Input: part model. Units: mm. Frame: model coordinates. Face numbers are marked on the shaded views. A direction names the side the tool comes from. Give positions to 0.01 mm unless a question says otherwise; leave off trailing zeros. Write each loop counter-clockwise with the first axis right and the second up, starting at its lowest first coordinate (ties: lowest second). Pieces come first, ordered by that corner, then holes. Notation, with made-up numbers: (79, 59) - (107, 59) arc R10 ccw to (107, 72) - close; hole circle Ø4 at (24.25, 48.5). An arc over 180 degrees is marked (long way). Answer as CSV lines item,"result".
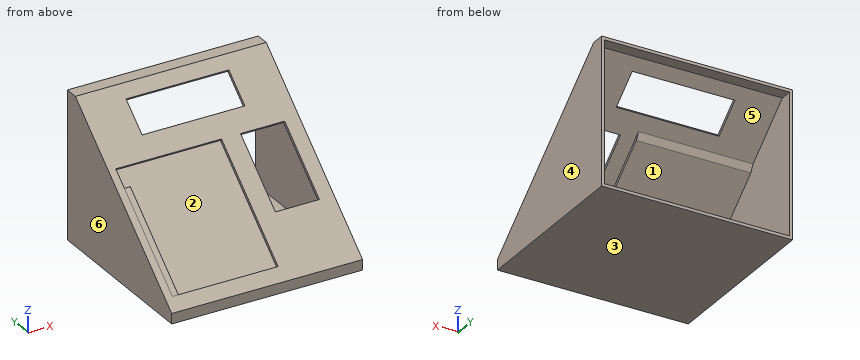
Solid Edge part; units mm, degrees
sketch "Sketch1" plane through (0, 0, 0) normal (0, 0, 1) x (1, 0, 0)
  line L0 (-65, -60) -> (65, -60)
  line L1 (65, -60) -> (65, 60)
  line L2 (65, 60) -> (-65, 60)
  line L3 (-65, 60) -> (-65, -60)
extrude "Protrusion1" add sketch "Sketch1" along normal blind 2
sketch "Sketch2" plane through (0, 0, 2) normal (0, 0, 1) x (1, 0, 0)
  line L0 (-65, -60) -> (-63, -60)
  line L1 (-63, -60) -> (-63, 60)
  line L2 (-63, 60) -> (-65, 60)
  line L3 (-65, 60) -> (-65, -60)
  line L4 (65, 60) -> (63, 60)
  line L5 (63, 60) -> (63, -60)
  line L6 (63, -60) -> (65, -60)
  line L7 (65, -60) -> (65, 60)
extrude "Protrusion2" add sketch "Sketch2" along normal blind 98
sketch "Sketch3" plane through (65, 0, 51) normal (1, 0, 0) x (0, 1, 0)
  line L0 (-60, 49) -> (-60, -44)
  line L1 (50.8331, 49) -> (-60, -44)
  line L2 (50.8331, 49) -> (-60, 49)
  dimension "D1" = 60
extrude "ExtrudedCutout_1" cut sketch "Sketch3" against normal blind 130
sketch "Sketch4" plane through (-63, 0, 52) normal (1, 0, 0) x (0, 1, 0)
  line L0 (-60, -45) -> (-60, -50)
  line L1 (-60, -50) -> (-58, -50)
  line L2 (-58, -50) -> (-58, -45.9326)
  line L3 (51.561, 46) -> (-58, -45.9326)
  line L4 (60, 46) -> (51.561, 46)
  line L5 (60, 48) -> (60, 46)
  line L6 (60, 48) -> (50.8331, 48)
  line L7 (50.8331, 48) -> (-60, -45)
extrude "Protrusion3" add sketch "Sketch4" along normal up to vertex (128 mm away)
sketch "Sketch5" plane through (0, -4.5835, 53.5) normal (0, -0.6427876, 0.7660444) x (1, 0, 0)
  line L0 (35, 62.3412) -> (-35, 62.3412)
  line L1 (-35, 62.3412) -> (-35, 38.3412)
  line L2 (-35, 38.3412) -> (35, 38.3412)
  line L3 (35, 38.3412) -> (35, 62.3412)
extrude "Cutout1" cut sketch "Sketch5" against normal blind 2
sketch "Sketch6" plane through (0, -4.5835, 53.5) normal (0, -0.6427876, 0.7660444) x (1, 0, 0)
  line L0 (-60, -62.3412) -> (12, -62.3412)
  line L1 (12, -62.3412) -> (12, 22.6588)
  line L2 (12, 22.6588) -> (-60, 22.6588)
  line L3 (-60, 22.6588) -> (-60, -62.3412)
  dimension "D1" = 12
  dimension "D2" = 12
extrude "ExtrudedCutout_3" cut sketch "Sketch6" against normal blind 2
sketch "Sketch7" plane through (0, -4.5835, 53.5) normal (0, -0.6427876, 0.7660444) x (1, 0, 0)
  line L0 (25, -29.5572) -> (55, -29.5572)
  line L1 (55, -29.5572) -> (55, 22.6588)
  line L2 (55, 22.6588) -> (25, 22.6588)
  line L3 (25, 22.6588) -> (25, -29.5572)
  dimension "D1" = 55
  dimension "D2" = 55
extrude "Cutout2" cut sketch "Sketch7" against normal blind 2
sketch "Sketch8" plane through (-63, 1, 50) normal (1, 0, 0) x (0, 1, 0)
  line L0 (14.3454, 15.0006) -> (-50.7684, -39.6363)
  line L1 (-55.8842, -41.3182) -> (-50.7684, -39.6363)
  line L2 (-52.054, -38.1042) -> (-55.8842, -41.3182)
  line L3 (-52.054, -38.1042) -> (13.0598, 16.5327)
  line L4 (13.0598, 16.5327) -> (16.89, 19.7467)
  line L5 (16.89, 19.7467) -> (14.3454, 15.0006)
extrude "ExtrudedProtrusion_6" add sketch "Sketch8" along normal blind 78
sketch "Sketch9" plane through (-60, -19.1399, 39.9803) normal (1, 0, 0) x (0, 0.7660444, 0.6427876)
  line L0 (-42.5, 1) -> (29.5, 1)
  line L1 (29.5, 1) -> (29.5, 0)
  line L2 (29.5, 0) -> (-42.5, 0)
  line L3 (-42.5, 0) -> (-42.5, 1)
extrude "ExtrudedProtrusion_7" add sketch "Sketch9" along normal blind 4
Item 1: Ray query, line 1 (X direction, y = 19.5, z = 47); line 2 (Z direction, x = -4, y = 54.5); line 3 (Z direction, x = -56, y = 20). Return the intervals inside material, ascending. Write a range as from..to.
The answers:
line 1,"-65..-63, 63..65"
line 2,"0..2, 98..100"
line 3,"0..2, 71.52..74.13"
Item 2: Mould query, pull axis X, two halves, no side actions, for the marked faces 1, 2, 3 and 4. Classes: +X half, -X half, draft (parallel to the pull), parting line (faces both ways), or undercut.
The answers:
face 1,"undercut"
face 2,"undercut"
face 3,"draft"
face 4,"+X half"
Item 3: Reachability of the marked faces 5 and 6 from +Z, -Z, +X, -X, +Y, -Y: full face, straight path, thin tool, end or side. Return the list, or none.
The answers:
face 5,"+Y"
face 6,"+Z, -Z, -X, +Y, -Y"
Item 4: Cut plane A-A on z = 90. Return the cut outline in (x, y).
The answers:
outline,"(-65, 38.92) - (-35, 38.92) - (-35, 42.03) - (-63, 42.03) - (-63, 60) - (-65, 60) - close; (35, 38.92) - (65, 38.92) - (65, 60) - (63, 60) - (63, 42.03) - (35, 42.03) - close"
Item 5: Cut plane C-C on y = -36.5. Return the cut outline in (x, z).
The answers:
outline,"(-65, 0) - (65, 0) - (65, 26.72) - (12, 26.72) - (12, 24.11) - (-60, 24.11) - (-60, 25.41) - (-56, 25.41) - (-56, 26.72) - (-65, 26.72) - close; hole (-63, 2) - (63, 2) - (63, 24.11) - (15, 24.11) - (15, 21.5) - (-63, 21.5) - close"
Item 6: Cut plane B-B on x = 40.5. Return the cut outline in (y, z).
The answers:
outline,"(-60, 0) - (60, 0) - (60, 2) - (-58, 2) - (-58, 6.07) - (-25.94, 32.97) - (-27.23, 34.5) - (-60, 7) - close; (12.77, 68.06) - (14.06, 66.53) - (51.56, 98) - (60, 98) - (60, 100) - (50.83, 100) - close"
Item 7: Contact query for flat-ended pins moving along their axis: pin 1 (8 mm diameter, centred on x = -9.5, z = 40.5, fed in from +Y); pin 2 (3 mm diameter, centred on x = 35.5, z = 20, fed in from -Y); pin 3 (1 mm diameter, centred on x = -37.5, z = 36.5, fed in from +Y). Output: stop coordinate, or through.
The answers:
pin 1,"y = -9.09"
pin 2,"y = -46.29"
pin 3,"y = -18.02"
Item 8: Cut plane D-D on z = 23.5. Return the cut outline in (x, y), plus the area to 3 significant figures.
The answers:
outline,"(-65, -40.34) - (-56, -40.34) - (-56, -38.78) - (-60, -38.78) - (-60, -37.22) - (12, -37.22) - (12, -40.34) - (65, -40.34) - (65, 60) - (63, 60) - (63, -37.22) - (15, -37.22) - (15, -34.11) - (-63, -34.11) - (-63, 60) - (-65, 60) - close"
area,"818 mm²"
